from build123d import *

# Parameters (mm, degrees)
CUT_EXTRUDE_1_DEPTH = 9
FILLET_1_R          = 0.4
CHAMFER_1_SIZE      = 5
CHAMFER_2_SIZE      = 5
SKETCH_5_W          = 18
SKETCH_5_H          = 74
CUT_EXTRUDE_2_DEPTH = 120
SKETCH_6_R          = 11
CUT_EXTRUDE_3_DEPTH = 54.05


with BuildPart() as part:
    # Эскиз1 → Повернуть1 (revolve)
    with BuildSketch(Plane(origin=(0, 0, 0), x_dir=(0, 0, -1), z_dir=(1, 0, 0))):
        Polygon((144, 0), (-122, 0), (-122, 42), (-37, 42), (-37, 60), (37, 60), (37, 42), (144, 42), align=None)
    revolve(axis=Axis((0, 0, 0), (0, 0, 1)))

    # Эскиз2 → Вырез-Вытянуть1 (cut)
    with BuildSketch(Plane(origin=(0, 42, 0), x_dir=(1, 0, 0), z_dir=(0, 1, 0))):
        with BuildLine():
            Line((-11, 67), (-11, 108))
            ThreePointArc((-11, 108), (0, 119), (11, 108))
            Line((11, 108), (11, 67))
            ThreePointArc((11, 67), (0, 56), (-11, 67))
        make_face()
    extrude(amount=-CUT_EXTRUDE_1_DEPTH, mode=Mode.SUBTRACT)

    # Скругление1
    fillet_1_edges = [part.edges().sort_by_distance(p)[0] for p in [
        (0, 33, -56),
        (-11, 33, -87.5),
        (0, 33, -119),
        (11, 33, -87.5),
    ]]
    fillet(fillet_1_edges, radius=FILLET_1_R)

    # Фаска1
    chamfer_1_edges = [part.edges().sort_by_distance(p)[0] for p in [
        (0, -42, -144),
    ]]
    chamfer(chamfer_1_edges, length=CHAMFER_1_SIZE)

    # Фаска2
    chamfer_2_edges = [part.edges().sort_by_distance(p)[0] for p in [
        (0, -42, 122),
    ]]
    chamfer(chamfer_2_edges, length=CHAMFER_2_SIZE)

    # Эскиз3 → Вырез-Повернуть1 (revolve, cut)
    with BuildSketch(Plane(origin=(0, 0, 0), x_dir=(0, 0, -1), z_dir=(1, 0, 0))):
        with BuildLine():
            Line((-37, 42), (-42, 42))
            Line((-42, 42), (-41, 41))
            Line((-41, 41), (-38.483239697, 41))
            ThreePointArc((-38.483239697, 41), (-37.588812506, 41.273350084), (-37, 42))
        make_face()
    revolve(axis=Axis((0, 0, 0), (0, 0, 1)), mode=Mode.SUBTRACT)

    # Эскиз5 → Вырез-Вытянуть2 (cut)
    with BuildSketch(Plane(origin=(0, 60, 0), x_dir=(1, 0, 0), z_dir=(0, 1, 0))):
        with Locations((-51, 0)):
            Rectangle(SKETCH_5_W, SKETCH_5_H)
        with Locations((51, 0)):
            Rectangle(SKETCH_5_W, SKETCH_5_H)
    extrude(amount=-CUT_EXTRUDE_2_DEPTH, mode=Mode.SUBTRACT)

    # Эскиз6 → Вырез-Вытянуть3 (cut)
    with BuildSketch(Plane(origin=(42, 0, 0), x_dir=(0, 0, -1), z_dir=(1, 0, 0))):
        Circle(SKETCH_6_R)
    extrude(amount=-CUT_EXTRUDE_3_DEPTH, mode=Mode.SUBTRACT)

    # Эскиз7 → Вырез-Повернуть6 (revolve, cut)
    with BuildSketch(Plane.XY):
        Polygon((-12.05, 11), (-12.05, 0), (-21.280095943, 0), align=None)
    revolve(axis=Axis((-21, 0, 0), (1, 0, 0)), mode=Mode.SUBTRACT)


solid = part.part
Design review of the part built by this model. Coordinates are the model's own, in mm. A direction names the side the tool comes from. Coordinates: 2 decimals unless noted, no trailing zeros. Write each loop counter-clockwise with the first axis right and the second up, starting at its lowest first coordinate (ties: lowest second). Pieces come first, ordered by that corner, then holes. Notation, with made-up numbers: (23, -25) -> (39, -25) arc R20 cw to (39, -9) -> close; hole circle Ø7 at (67.5, 3). An arc over 180 degrees is marked (long way). Write each question's results on one line, items separated by ' | '. Start each with the question number.
(1) Take a section at D-D on z = -21.5. Write out the cut boundary in (x, y).
(2) Take a section at B-B on z = -86. Write out the cut boundary in (x, y).
(3) Tool access review of faces 1 (the face through (15.35, -10.74, 2.38)), 2 (the face through (0, -46, -37)), 3 (the face through (-11, 37, -87)): name each direction out of +Z, -Z, +X, -X, +Y, -Y from which nothing blocks a thin tool from reaching the whole face with its end or side.
(4) Take a section at C-C on z = 97.5. Write out the cut boundary in (x, y).
(5) The part is to be moulded in two halves that separate along X. For faces 4 (the face through (33.041, 17.185, 121.757)), 5 (the face through (-19.68, 1.82, 0.57)), 6 (the face through (11, 37, -88)), say which applies: pulls with the +X half, pulls with the -X half, needs draft (parallel to the pull), parting line crosses it, or undercut.
(6) Clearance check with flat-ended pins moving along their axes: P1, Ø4, axis at x = -30.5, z = -33, coming from the -Y side; P2, Ø8, axis at y = 36, z = -92.5, coming from the -X side; P3, Ø1, axis at x = 33, z = -73, coming from the -Y side. State where each tip first meets the part, or that it passes through.
(7) For line 1 along Z through (x, y) = (8, 0); line 2 along Y through (x, z) = (15, 0); line 3 along Z through (x, y) = (11.5, 1.5), list the stretches that pass through material, from the lowest coordinate up. Write a range as from..to.
Results found:
1) outline: (-42, -42.85) arc R60 ccw to (42, -42.85) -> (42, 42.85) arc R60 ccw to (-42, 42.85) -> close
2) outline: (-11, 33.4) -> (-11, 40.53) arc R42 ccw (long way) to (11, 40.53) -> (11, 33.4) arc R0.4 cw to (10.6, 33) -> (-10.6, 33) arc R0.4 cw to start
3) face 1: +X | face 2: -Z, -Y | face 3: +Y
4) outline: circle Ø84 at (0, 0)
5) face 4: parting line crosses it | face 5: pulls with the +X half | face 6: undercut
6) P1: stops at y = -52.8 | P2: stops at x = -27.2 | P3: stops at y = -26.6
7) line 1: z = -144..-11, 11..122 | line 2: y = -58.09..-11, 11..58.09 | line 3: z = -144..-10.9, 10.9..122
